from build123d import *


with BuildPart() as part:
    # Эскиз1 → Повернуть1 (revolve)
    with BuildSketch(Plane.XY):
        with BuildLine():
            Line((0, 11), (0, 0))
            Line((0, 0), (5, 0))
            ThreePointArc((5, 0), (7.121320344, 0.878679656), (8, 3))
            ThreePointArc((8, 3), (10.2627417, 3.9372583), (11.2, 6.2))
            ThreePointArc((11.2, 6.2), (28, 7.8), (44.8, 6.2))
            ThreePointArc((44.8, 6.2), (45.7372583, 3.9372583), (48, 3))
            Line((48, 3), (51, 3))
            Line((51, 3), (51, 7))
            Line((51, 7), (59.457233587, 3.92181871))
            ThreePointArc((59.457233587, 3.92181871), (62.204023326, 4.28344044), (63.483294017, 6.740896572))
            Line((63.483294017, 6.740896572), (63.483294017, 8.174747022))
            ThreePointArc((63.483294017, 8.174747022), (63.342755698, 8.808674415), (62.947475432, 9.323813687))
            Line((62.947475432, 9.323813687), (60.949874371, 11))
            Line((60.949874371, 11), (0, 11))
        make_face()
    revolve(axis=Axis((0, 11, 0), (1, 0, 0)))


solid = part.part
Verification items for the finished model (mm, model axes). A direction names the side the tool comes from. Coordinates: 2 decimals unless noted, no trailing zeros. Order: outer loops, then holes, each group sorted by start corner. A loop starts at its lowest first (then second) coordinate and runs counter-clockwise, first axis right, second up.
1. Go/stop test with flat-tipped pins: pin 1 Ø12 at (x, z) = (8, -5.5) entering from -Y; pin 2 Ø5 at (x, z) = (25.5, 7) entering from -Y; pin 3 Ø1 at (x, z) = (7, -0.5) entering from +Y; pin 4 Ø10 at (x, z) = (29, 4.5) entering from -Y. Record where each tip stops, or that it passes through.
Results found:
pin 1: stops at y = 0
pin 2: passes through
pin 3: stops at y = 21.59
pin 4: stops at y = 7.74
2. Release check for a two-part mould opening along Z. For faces 4 (the face through (2.535, 0.839, 4.213)), 5 (the face through (51, 9, -4)), 6 (the face through (61.49, 10.58, 0.17)) record: +Z half, -Z half, draft (parallel to the pull), parting line (faces both ways), or undercut.
Results found:
face 4: parting line
face 5: draft
face 6: undercut
3. Set-up check for faces 1 (the face through (49.52, 12.73, 7.81)), 2 (the face through (0, 11, 0)), 3 (the face through (53.408, 6.495, 1.868)): record each of +Z, -Z, +X, -X, +Y, -Y from which the full face is reachable in a straight line by a thin tool's end or side.
Results found:
face 1: +X
face 2: +Z, -Z, -X, +Y, -Y
face 3: none
4. Sectioned sample at A-A, the plane x = 53.5. Record the cut outline in (y, z), and give its area (3 significant figures).
Results found:
outline: circle Ø9.82 at (11, 0)
area: 75.7 mm2
5. Sectioned sample at B-B, the plane x = 47. Record the cut outline in (y, z), and give its area (3 significant figures).
Results found:
outline: circle Ø15.68 at (11, 0)
area: 193 mm2
6. Scan lines: line 1 (X direction, y = 13.5, z = 4.5); line 2 (X direction, y = 7.5, z = -6.5); line 3 (Z direction, x = 50.5, y = 11.25). Record each from-to range of solid material in increasing order.
Results found:
line 1: x = 0 to 11.18, 44.82 to 51, 54.15 to 63.35
line 2: x = 0 to 9.89, 46.11 to 51
line 3: z = -8 to 8
